Verification items for this drawing (mm, ordinates from the low corner). A direction names the side the tool comes from. Give positions to 0.01 mm unless a question says otherwise; leave off trailing zeros. Loops run counter-clockwise (first coordinate to the right, second up) from the corner with the lowest first, then second, coordinate; pieces in that order, holes last. Notation, with made-up numbers: (26, 22) -> (33, 22) arc R12 cw to (33, 42) -> close; hole circle Ø4 at (46.5, -35). An arc over 180 degrees is marked (long way). Write each question's results on one line, items separated by ' | '. Start each with the question number.
Item 1: Cross-section at C-C on z = 69. Enter the section's corners in (x, y).
Item 2: Access from +Z, -Z, +X, -X, +Y, -Y to the whole of each face (thin tool, end or side, straight path). Record for the marked faces 1 and 2.
Item 3: Gauge pin test, flat ends, axial feed: pin 1 Ø4 at (x, y) = (17.5, 15.5) entering from -Z; pin 2 Ø5 at (y, z) = (6, 24) entering from -X; pin 3 Ø2 at (x, y) = (25.5, 15.5) entering from +Z; pin 4 Ø5 at (x, z) = (23, 25) entering from -Y. Record the tip position at first contact, or that the pin passes through.
Item 4: Cross-section at A-A on y = 25. Enter the section's corners in (x, z).
Item 5: Cross-section at B-B on x = 25. Enter the section's corners in (y, z).
Item 6: Cross-section at D-D on z = 60. Enter the section's corners in (x, y).
Item 7: Scan lines: line 1 along Z through (x, y) = (25, 26); line 2 along X through (y, z) = (24, 11); line 3 along Z through (x, y) = (41.5, 38.5). Record each from-to range of solid material in increasing order.
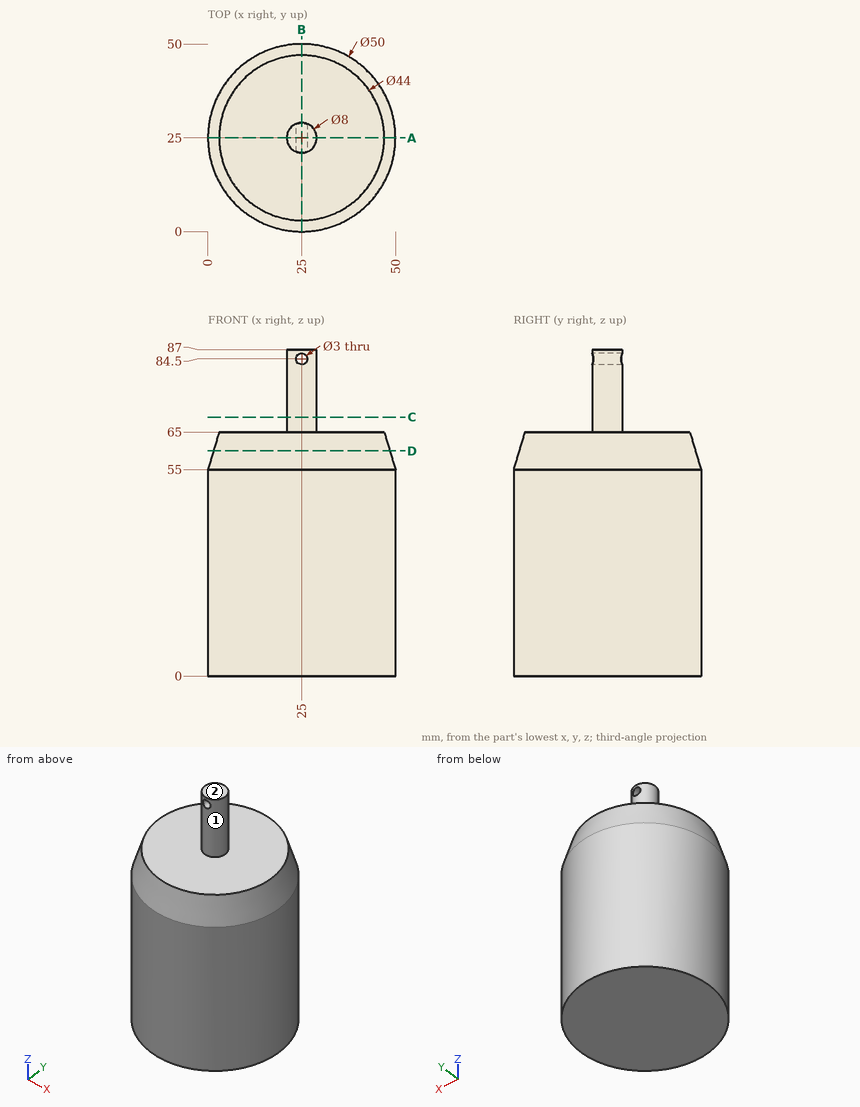
Answer sheet:
1) outline: circle Ø8 at (25, 25)
2) face 1: +Z | face 2: +Z, +X, -X, +Y, -Y
3) pin 1: stops at z = 0 | pin 2: stops at x = 6.22 | pin 3: stops at z = 65 | pin 4: stops at y = 0
4) outline: (0, 0) -> (50, 0) -> (50, 55) -> (47, 65) -> (29, 65) -> (29, 87) -> (21, 87) -> (21, 65) -> (3, 65) -> (0, 55) -> close; hole circle Ø3 at (25, 84.5)
5) outline: (0, 0) -> (50, 0) -> (50, 55) -> (47, 65) -> (29, 65) -> (29, 83) -> (21, 83) -> (21, 65) -> (3, 65) -> (0, 55) -> close; (21, 86) -> (29, 86) -> (29, 87) -> (21, 87) -> close
6) outline: circle Ø47 at (25, 25)
7) line 1: z = 0 to 83, 86 to 87 | line 2: x = 0.02 to 49.98 | line 3: z = 0 to 65
